```python
from build123d import *

# Parameters (mm, degrees)
F0_W     = 20
F0_H     = 30
F1_DEPTH = 3
F3_DEPTH = 1
F5_DEPTH = 0.2


with BuildPart() as f1:
    # F0 (on Top) → F1 (new body)
    with BuildSketch(Plane.XY):
        with Locations((10, 28.513513)):
            Rectangle(F0_W, F0_H)
    extrude(amount=F1_DEPTH)

    # F2 (on face) → F3 (join)
    with BuildSketch(Plane.XY.offset(3)):
        Polygon((19.342611, 41.524556), (17.694369, 43.052193), (2.056164, 43.052193), (0.689328, 41.577448), (0.689328, 31.836104), (2.122905, 30.507424), (2.122905, 28.821025), (0.744304, 27.333586), (0.698527, 16.487885), (2.982544, 14.308448), (17.446602, 14.308448), (19.342611, 16.442662), (19.342611, 27.333586), (18.056178, 28.821025), (18.056178, 30.54967), (19.342611, 31.836104), align=None)
    extrude(amount=F3_DEPTH)

    # F4 (on face) → F5 (join)
    with BuildSketch(Plane.XY.offset(3)):
        with BuildLine():
            Line((19.270148, 42.736807), (19.582438, 42.736807))
            ThreePointArc((19.582438, 42.736807), (19.485372, 42.970235), (19.270148, 43.102861))
            Line((19.270148, 43.102861), (19.270148, 42.736807))
        make_face()
        with BuildLine():
            Line((19.107276, 42.736807), (19.107276, 43.109485))
            ThreePointArc((19.107276, 43.109485), (18.870383, 42.982736), (18.762206, 42.736807))
            Line((18.762206, 42.736807), (19.107276, 42.736807))
        make_face()
        with BuildLine():
            Line((0.654074, 42.812039), (0.654074, 43.161998))
            ThreePointArc((0.654074, 43.161998), (0.429915, 43.042523), (0.323149, 42.812039))
            Line((0.323149, 42.812039), (0.654074, 42.812039))
        make_face()
        with BuildLine():
            Line((0.807343, 42.812039), (1.117002, 42.812039))
            ThreePointArc((1.117002, 42.812039), (1.017574, 43.03455), (0.807343, 43.157838))
            Line((0.807343, 43.157838), (0.807343, 42.812039))
        make_face()
        with BuildLine():
            ThreePointArc((0.807343, 42.378449), (1.001335, 42.484646), (1.109067, 42.67779))
            Line((1.109067, 42.67779), (0.807343, 42.67779))
            Line((0.807343, 42.67779), (0.807343, 42.378449))
        make_face()
        with BuildLine():
            ThreePointArc((0.331085, 42.67779), (0.446612, 42.47712), (0.654074, 42.374289))
            Line((0.654074, 42.374289), (0.654074, 42.67779))
            Line((0.654074, 42.67779), (0.331085, 42.67779))
        make_face()
        with BuildLine():
            ThreePointArc((18.766535, 42.634873), (18.882517, 42.411034), (19.107276, 42.296845))
            Line((19.107276, 42.296845), (19.107276, 42.634873))
            Line((19.107276, 42.634873), (18.766535, 42.634873))
        make_face()
        with BuildLine():
            ThreePointArc((19.270148, 42.303468), (19.473758, 42.423052), (19.578109, 42.634873))
            Line((19.578109, 42.634873), (19.270148, 42.634873))
            Line((19.270148, 42.634873), (19.270148, 42.303468))
        make_face()
        with BuildLine():
            Line((0.996978, 29.684267), (1.370052, 29.684267))
            ThreePointArc((1.370052, 29.684267), (1.252467, 29.951603), (0.996978, 30.093093))
            Line((0.996978, 30.093093), (0.996978, 29.684267))
        make_face()
        with BuildLine():
            Line((0.838792, 29.684267), (0.838792, 30.094109))
            ThreePointArc((0.838792, 30.094109), (0.579506, 29.953764), (0.459937, 29.684267))
            Line((0.459937, 29.684267), (0.838792, 29.684267))
        make_face()
        with BuildLine():
            ThreePointArc((0.468405, 29.547278), (0.599281, 29.31341), (0.838792, 29.193174))
            Line((0.838792, 29.193174), (0.838792, 29.547278))
            Line((0.838792, 29.547278), (0.468405, 29.547278))
        make_face()
        with BuildLine():
            ThreePointArc((0.996978, 29.19419), (1.232823, 29.315445), (1.361583, 29.547278))
            Line((1.361583, 29.547278), (0.996978, 29.547278))
            Line((0.996978, 29.547278), (0.996978, 29.19419))
        make_face()
        with BuildLine():
            Line((19.202649, 29.588132), (19.539459, 29.588132))
            ThreePointArc((19.539459, 29.588132), (19.430045, 29.827535), (19.202649, 29.960107))
            Line((19.202649, 29.960107), (19.202649, 29.588132))
        make_face()
        with BuildLine():
            Line((19.050451, 29.588132), (19.050451, 29.966929))
            ThreePointArc((19.050451, 29.966929), (18.79808, 29.84169), (18.67526, 29.588132))
            Line((18.67526, 29.588132), (19.050451, 29.588132))
        make_face()
        with BuildLine():
            ThreePointArc((18.683212, 29.437403), (18.814648, 29.21315), (19.050451, 29.103779))
            Line((19.050451, 29.103779), (19.050451, 29.437403))
            Line((19.050451, 29.437403), (18.683212, 29.437403))
        make_face()
        with BuildLine():
            ThreePointArc((19.202649, 29.1106), (19.414205, 29.226579), (19.531507, 29.437403))
            Line((19.531507, 29.437403), (19.202649, 29.437403))
            Line((19.202649, 29.437403), (19.202649, 29.1106))
        make_face()
        with BuildLine():
            Line((0.994411, 14.655351), (0.994411, 15.033354))
            ThreePointArc((0.994411, 15.033354), (0.747631, 14.904186), (0.622466, 14.655351))
            Line((0.622466, 14.655351), (0.994411, 14.655351))
        make_face()
        with BuildLine():
            Line((1.184542, 14.655351), (1.521054, 14.655351))
            ThreePointArc((1.521054, 14.655351), (1.408339, 14.891019), (1.184542, 15.025773))
            Line((1.184542, 15.025773), (1.184542, 14.655351))
        make_face()
        with BuildLine():
            ThreePointArc((1.184542, 14.14473), (1.408339, 14.279484), (1.521054, 14.515152))
            Line((1.521054, 14.515152), (1.184542, 14.515152))
            Line((1.184542, 14.515152), (1.184542, 14.14473))
        make_face()
        with BuildLine():
            ThreePointArc((0.622466, 14.515152), (0.747631, 14.266317), (0.994411, 14.137149))
            Line((0.994411, 14.137149), (0.994411, 14.515152))
            Line((0.994411, 14.515152), (0.622466, 14.515152))
        make_face()
        with BuildLine():
            Line((19.278564, 14.661851), (19.591466, 14.655351))
            ThreePointArc((19.591466, 14.655351), (19.48198, 14.86364), (19.278564, 14.981936))
            Line((19.278564, 14.981936), (19.278564, 14.661851))
        make_face()
        with BuildLine():
            Line((19.113579, 14.665279), (19.113579, 14.990424))
            ThreePointArc((19.113579, 14.990424), (18.889292, 14.885036), (18.761711, 14.672588))
            Line((18.761711, 14.672588), (19.113579, 14.665279))
        make_face()
        with BuildLine():
            ThreePointArc((18.752394, 14.515152), (18.871129, 14.270688), (19.113579, 14.147892))
            Line((19.113579, 14.147892), (19.113579, 14.515152))
            Line((19.113579, 14.515152), (18.752394, 14.515152))
        make_face()
        with BuildLine():
            ThreePointArc((19.278564, 14.15638), (19.493042, 14.286674), (19.596844, 14.515152))
            Line((19.596844, 14.515152), (19.278564, 14.515152))
            Line((19.278564, 14.515152), (19.278564, 14.15638))
        make_face()
    extrude(amount=F5_DEPTH)


solid = f1.part
```
Part model, mm, in its own coordinate system. A direction names the side the tool comes from. Round coordinates to 2 decimals unless told otherwise and drop trailing zeros. Write each loop counter-clockwise with the first axis right and the second up, starting at its lowest first coordinate (ties: lowest second). Pieces come first, ordered by that corner, then holes. Notation, with made-up numbers: (18, -4) -> (55, -4) arc R26 ccw to (55, 25) -> close; hole circle Ø3 at (23, 15.5). An arc over 180 degrees is marked (long way). Return JSON: item names as keys, results as strings. Group by question number.
Q1. Saw through at A-A on y = 18.5. Write the cut outline in (x, z).
Q2. Probe L1, parallel to X at y = 39, z = 3.75; L2, parallel to Y at x = 12.25, z = 3.7; L3, parallel to X at y = 42, z = 3.6. List the from-to ranges inside material, lowest first. Write a range as [from, to].
Q3. Pin check, flat tips, straight feed: pin 1 (0.5 mm diameter, centred on y = 37, z = 3.5, fed in from -X); pin 2 (0.8 mm diameter, centred on x = 7, z = 3.5, fed in from +Y); pin 3 (0.8 mm diameter, centred on y = 29.5, z = 3.5, fed in from -X). Stop position of each tip, or through.
Q4. Mould opens along X. For faces 5 (the flat face through (18.69, 31.184, 3.493)), 6 (the flat face through (10, 29, 4)), 7 (the flat face through (10, 43.052, 3.5)) say: pulls with the +X half, pulls with the -X half, needs draft (parallel to the pull), parting line crosses it, or undercut.
Q5. Saw through at C-C on y = 25. Write the cut outline in (x, z), plus the area to 3 significant figures.
Q6. Which spindle directions (+Z, -Z, +X, -X, +Y, -Y) get a long thin tool onto all of the face, cutting with end or side? Do faces 1 (the flat face through (10, 29, 0)), 2 (the flat face through (18.708, 28.067, 3.493)), 3 (the flat face through (0.689, 36.8, 3.5)), 4 (the flat face through (10.1, 14.308, 3.5)). Say none if no direction does.
Q7. Saw through at B-B on z = 3.5. Write the cut outline in (x, y), plus the area to 3 significant figures.
Answer:
{
 "1": {"outline": "(0, 0) -> (20, 0) -> (20, 3) -> (19.34, 3) -> (19.34, 4) -> (0.71, 4) -> (0.71, 3) -> (0, 3) -> close"},
 "2": {"L1": "[0.69, 19.34]", "L2": "[14.31, 43.05]", "L3": "[1.08, 18.83]"},
 "3": {"pin 1": "x = 0.69", "pin 2": "y = 43.05", "pin 3": "x = 0.46"},
 "4": {"face 5": "pulls with the +X half", "face 6": "needs draft", "face 7": "undercut"},
 "5": {"outline": "(0, 0) -> (20, 0) -> (20, 3) -> (19.34, 3) -> (19.34, 4) -> (0.73, 4) -> (0.73, 3) -> (0, 3) -> close", "area": "78.6 mm2"},
 "6": {"face 1": "-Z, +X, -X, +Y, -Y", "face 2": "+Z, +X", "face 3": "+Z, -X, +Y", "face 4": "+Z, -Y"},
 "7": {"outline": "(0.69, 31.84) -> (2.12, 30.51) -> (2.12, 28.82) -> (0.74, 27.33) -> (0.7, 16.49) -> (2.98, 14.31) -> (17.45, 14.31) -> (19.34, 16.44) -> (19.34, 27.33) -> (18.06, 28.82) -> (18.06, 30.55) -> (19.34, 31.84) -> (19.34, 41.52) -> (17.69, 43.05) -> (2.06, 43.05) -> (0.69, 41.58) -> close", "area": "521 mm2"}
}
